For this review, use the dimensioned drawing (mm, ordinates from the lowest corner) and the shaded views. A direction names the side the tool comes from. Give positions to 0.01 mm unless a question says otherwise; leave off trailing zeros. Write each loop counter-clockwise with the first axis right and the second up, starting at its lowest first coordinate (ties: lowest second). Pieces come first, ordered by that corner, then holes. Notation, with made-up numbers: M 88,65.25 L 97,65.25 A8 cw 97,78.25 Z; hole C -26.5,19 d1. An arc over 180 degrees is marked long. Answer in a Markdown table with one row per item.
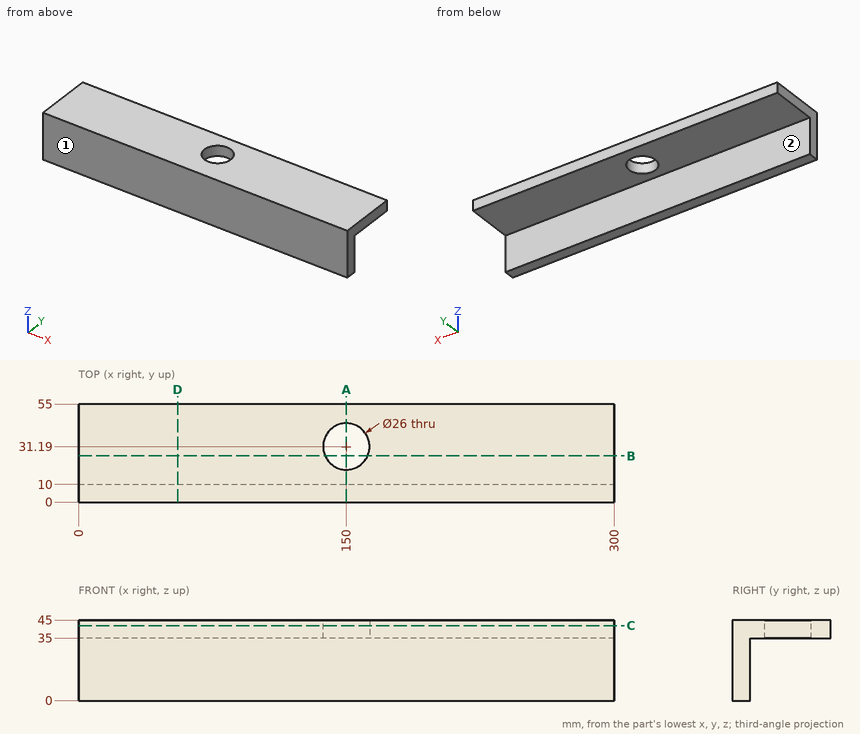
1) Add section D-D (x = 55.5). Write out the cut boundary in (y, z), and give its area (3 significant figures).
Geometry says:
| item | result |
|---|---|
| outline | M 0,0 L 10,0 L 10,35 L 55,35 L 55,45 L 0,45 Z |
| area | 900 mm^2 |
2) Add section C-C (z = 42). Write out the cut boundary in (x, y), and give its area (3 significant figures).
Geometry says:
| item | result |
|---|---|
| outline | M 0,0 L 300,0 L 300,55 L 0,55 Z; hole C 150,31.19 d26 |
| area | 16,000 mm^2 |
3) To check wall thickness, follow probe 1 along Y at (x, z) = (150, 40); probe 2 along Y at (x, z) = (217.5, 16.5); probe 3 along Z at (x, y) = (247, 24.5). State the ranges of each line that lie inside material, in increasing order. Write a range as [from, to].
Geometry says:
| item | result |
|---|---|
| probe 1 | [0, 18.19], [44.19, 55] |
| probe 2 | [0, 10] |
| probe 3 | [35, 45] |
4) Add section A-A (x = 150). Write out the cut boundary in (y, z), and give its area (3 significant figures).
Geometry says:
| item | result |
|---|---|
| outline | M 0,0 L 10,0 L 10,35 L 18.19,35 L 18.19,45 L 0,45 Z; M 44.19,35 L 55,35 L 55,45 L 44.19,45 Z |
| area | 640 mm^2 |
5) Add section B-B (y = 26). Write out the cut boundary in (x, z).
Geometry says:
| item | result |
|---|---|
| outline | M 0,35 L 138.08,35 L 138.08,45 L 0,45 Z; M 161.92,35 L 300,35 L 300,45 L 161.92,45 Z |
6) Insertion check: P1, Ø1, axis at x = 248, z = 30.5, coming from the +Y side; P2, Ø1.5, axis at x = 172.5, y = 24.5, coming from the -Z side. Each pin has a flat end and moves straight along its axis. Give the tip position at first contact, or say it passes through.
Geometry says:
| item | result |
|---|---|
| P1 | y = 10 |
| P2 | z = 35 |
7) For the marked faces 1 and 2, list the 3-axis set-ups (+Z, -Z, +X, -X, +Y, -Y) from which the entire face can be reached by the end or side of a thin tool; tool diameter is ignored.
Geometry says:
| item | result |
|---|---|
| face 1 | +Z, -Z, +X, -X, -Y |
| face 2 | -Z, +X, -X, +Y |
